```python
from build123d import *

# Parameters (mm, degrees)
BOSS_EXTRUDE1_DEPTH = 39.624
SKETCH2_R           = 2.5527
CUT_EXTRUDE1_DEPTH  = 41.236833499


with BuildPart() as part:
    # Sketch1 → Boss-Extrude1 (new body)
    with BuildSketch(Plane(origin=(0, 0, 0), x_dir=(1, 0, 0), z_dir=(0, 1, 0))):
        with BuildLine():
            Line((-0.742977689, 5.070302945), (-4.019522311, 3.178589026))
            ThreePointArc((-4.019522311, 3.178589026), (-4.43790388, 2.562225), (-4.7625, 1.891713919))
            Line((-4.7625, 1.891713919), (-4.7625, -1.891713919))
            ThreePointArc((-4.7625, -1.891713919), (-4.43790388, -2.562225), (-4.019522311, -3.178589026))
            Line((-4.019522311, -3.178589026), (-0.742977689, -5.070302945))
            ThreePointArc((-0.742977689, -5.070302945), (0, -5.12445), (0.742977689, -5.070302945))
            Line((0.742977689, -5.070302945), (4.019522311, -3.178589026))
            ThreePointArc((4.019522311, -3.178589026), (4.43790388, -2.562225), (4.7625, -1.891713919))
            Line((4.7625, -1.891713919), (4.7625, 1.891713919))
            ThreePointArc((4.7625, 1.891713919), (4.43790388, 2.562225), (4.019522311, 3.178589026))
            Line((4.019522311, 3.178589026), (0.742977689, 5.070302945))
            ThreePointArc((0.742977689, 5.070302945), (0, 5.12445), (-0.742977689, 5.070302945))
        make_face()
    extrude(amount=BOSS_EXTRUDE1_DEPTH)

    # Sketch2 → Cut-Extrude1 (cut, through all)
    with BuildSketch(Plane(origin=(0, 39.624, 0), x_dir=(1, 0, 0), z_dir=(0, 1, 0))):
        with Locations(Location((0, 0, 0), (0, 0, 270))):
            Circle(SKETCH2_R)
    extrude(amount=-CUT_EXTRUDE1_DEPTH, mode=Mode.SUBTRACT)


solid = part.part
```
Can you work these out from the model? Positions are in its coordinate system, mm. Coordinates: 2 decimals unless noted, no trailing zeros. Order: outer loops, then holes, each group sorted by start corner. A loop starts at its lowest first (then second) coordinate and runs counter-clockwise, first axis right, second up.
1. If we section it at A-A (z = 0): Please give me the cut outline in (x, y), then the cut area to 3 significant figures.
2. I'm going to push flat-ended pins straight in: pin 1 (1 mm diameter, centred on x = 3.5, y = 4.5, fed in from -Z); pin 2 (1 mm diameter, centred on x = -3.5, y = 9.5, fed in from +Z). Where does each tip first touch, or does it pass through?
3. If we section it at D-D (z = 4): Please give me the cut outline in (x, y).
4. If we section it at C-C (x = 0): Please give me the cut outline in (y, z).
5. Thinking about a two-plate mould opening in X: for faces 1 (the face through (0.767, 20.089, 2.435)), 2 (the face through (4.443, 19.535, -2.553)), 3 (the face through (-4.443, 19.535, 2.553)), 4 (the face through (-2, 0, -2)), which applies, +X half, -X half, draft (parallel to the pull), parting line (faces both ways), or undercut?
6. If we section it at B-B (y = 5): Please give me the cut outline in (x, z).
7. I need wall thicknesses on line 1 (X direction, y = 18.5, z = 0); line 2 (Z direction, x = 0.5, y = 26); line 3 (Z direction, x = 1, y = 28). Which ranges of each line are inside material? Lowest first, please.
Entries:
1. outline: (-4.76, 0) - (-2.55, 0) - (-2.55, 39.62) - (-4.76, 39.62) - close; (2.55, 0) - (4.76, 0) - (4.76, 39.62) - (2.55, 39.62) - close
1. area: 175 mm2
2. pin 1: stops at z = -3.77
2. pin 2: stops at z = 3.77
3. outline: (-2.6, 0) - (2.6, 0) - (2.6, 39.62) - (-2.6, 39.62) - close
4. outline: (0, -5.12) - (39.62, -5.12) - (39.62, -2.55) - (0, -2.55) - close; (0, 2.55) - (39.62, 2.55) - (39.62, 5.12) - (0, 5.12) - close
5. face 1: undercut
5. face 2: +X half
5. face 3: -X half
5. face 4: draft
6. outline: (-4.76, -1.89) arc R5.12 ccw to (-4.02, -3.18) - (-0.74, -5.07) arc R5.12 ccw to (0.74, -5.07) - (4.02, -3.18) arc R5.12 ccw to (4.76, -1.89) - (4.76, 1.89) arc R5.12 ccw to (4.02, 3.18) - (0.74, 5.07) arc R5.12 ccw to (-0.74, 5.07) - (-4.02, 3.18) arc R5.12 ccw to (-4.76, 1.89) - close; hole circle Ø5.11 at (0, 0)
7. line 1: x = -4.76 to -2.55, 2.55 to 4.76
7. line 2: z = -5.1 to -2.5, 2.5 to 5.1
7. line 3: z = -4.92 to -2.35, 2.35 to 4.92
